Build history of the part. All positions in model axes, mm. Face numbers are marked on the shaded views. A direction names the side the tool comes from. Give positions to 0.01 mm unless a question says otherwise; leave off trailing zeros. Order: outer loops, then holes, each group sorted by start corner. A loop starts at its lowest first (then second) coordinate and runs counter-clockwise, first axis right, second up. Notation, with made-up numbers: (80, 83) -> (129, 83) arc R5 ccw to (129, 90) -> close; hole circle Ø8 at (19, 12). An arc over 180 degrees is marked (long way). Use a Markdown table: item, result. Add a question column.
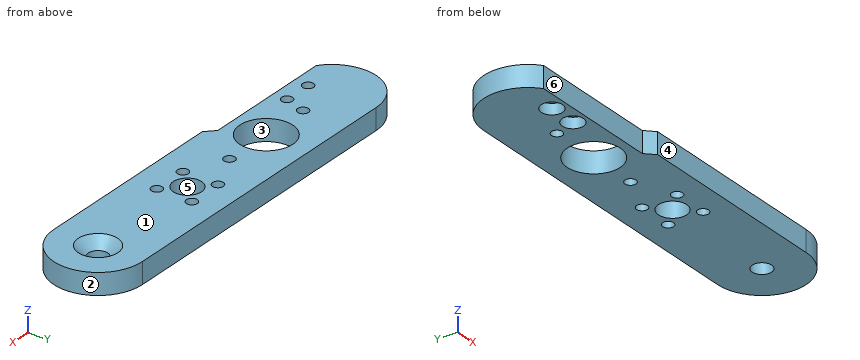
```python
from build123d import *

# Parameters (mm, degrees)
SKETCH2_R                     = 4
SKETCH2_R_2                   = 1.55
SKETCH2_R_3                   = 7.5
BOSS_EXTRUDE1_DEPTH           = 6
CSK_FOR_M5_SFHCS1_D           = 5.5
CSK_FOR_M5_SFHCS1_CSINK_D     = 11.2
CSK_FOR_M5_SFHCS1_CSINK_ANGLE = 90
SKETCH6_R                     = 1.55
CUT_EXTRUDE1_DEPTH            = 3
SKETCH7_R                     = 3
CUT_EXTRUDE2_DEPTH            = 59.49909717


with BuildPart() as part:
    # Sketch2 → Boss-Extrude1 (new body)
    with BuildSketch(Plane.XY):
        with BuildLine():
            Line((-44.569206843, 12.5), (44.430793157, 12.5))
            ThreePointArc((44.430793157, 12.5), (56.930793157, 0), (44.430793157, -12.5))
            Line((44.430793157, -12.5), (-12.069206843, -12.5))
            Line((-12.069206843, -12.5), (-14.569206843, -10))
            Line((-14.569206843, -10), (-52.069206843, -10))
            ThreePointArc((-52.069206843, -10), (-56.427748069, 3.952847075), (-44.569206843, 12.5))
        make_face()
        with Locations((10.430793157, 0)):
            Circle(SKETCH2_R, mode=Mode.SUBTRACT)
        with Locations((15.380540625, 4.949747468)):
            Circle(SKETCH2_R_2, mode=Mode.SUBTRACT)
        with Locations((15.380540625, -4.949747468)):
            Circle(SKETCH2_R_2, mode=Mode.SUBTRACT)
        with Locations((5.481045689, -4.949747468)):
            Circle(SKETCH2_R_2, mode=Mode.SUBTRACT)
        with Locations((5.481045689, 4.949747468)):
            Circle(SKETCH2_R_2, mode=Mode.SUBTRACT)
        with Locations((-19.569206843, 0)):
            Circle(SKETCH2_R_3, mode=Mode.SUBTRACT)
        with Locations((-5.569206843, 0)):
            Circle(SKETCH2_R_2, mode=Mode.SUBTRACT)
        with Locations((-33.569206843, 0)):
            Circle(SKETCH2_R_2, mode=Mode.SUBTRACT)
    extrude(amount=BOSS_EXTRUDE1_DEPTH)

    # CSK for M5 SFHCS1 (through all)
    with Locations(Plane(origin=(44.430793157, 0, 6), x_dir=(1, 0, 0), z_dir=(0, 0, 1))):
        with Locations((0, 0)):
            CounterSinkHole(CSK_FOR_M5_SFHCS1_D / 2, CSK_FOR_M5_SFHCS1_CSINK_D / 2, counter_sink_angle=CSK_FOR_M5_SFHCS1_CSINK_ANGLE)

    # Sketch6 → Cut-Extrude1 (cut)
    with BuildSketch(Plane.XY.offset(6)):
        with Locations((-35.569206843, -6)):
            Circle(SKETCH6_R)
        with Locations((-43.569206843, -6)):
            Circle(SKETCH6_R)
    extrude(amount=-CUT_EXTRUDE1_DEPTH, mode=Mode.SUBTRACT)

    # Sketch7 → Cut-Extrude2 (cut, through all)
    with BuildSketch(Plane.XY.offset(3)):
        with Locations((-35.569206843, -6)):
            Circle(SKETCH7_R)
        with Locations((-43.569206843, -6)):
            Circle(SKETCH7_R)
    extrude(amount=-CUT_EXTRUDE2_DEPTH, mode=Mode.SUBTRACT)


solid = part.part
```
(1) Wall check: probe 1 along X at (y, z) = (1.25, 5.25); probe 2 along X at (y, z) = (1, 4.55); probe 3 along Y at (x, z) = (12.5, 4.1). Give the ranges that are in metal, low to high.
(2) Mould opens along Y. For the marked faces 1, 2, 3 and 4 say: released by +Y, released by -Y, zero draft, split by the parting line, or undercut.
(3) Band-saw the part on D-D on y = 10.5. Give the cut face in (x, z), plus the area to 3 significant figures.
(4) Pin check, flat tips, straight feed: pin 1 Ø3 at (x, y) = (-44.5, -5) entering from -Z; pin 2 Ø1.8 at (x, z) = (-27.5, 3.5) entering from -Y. Stop position of each tip, or through.
(5) Band-saw the part on B-B on x = 11.5. Give the cut face in (y, z).
(6) Band-saw the part on A-A on y = 0. Give the cut face in (x, z), plus the area to 3 significant figures.
(7) Tool access for the marked faces 5 and 6: list every direction of +Z, -Z, +X, -X, +Y, -Y with a clear straight run to the whole face (end or side of a thin tool).
(8) Band-saw the part on C-C on z = 4.2. State how many separate pieces and enclosed holes the cut face has, plus the area to 3 significant figures.
Response:
| question | item | result |
|---|---|---|
| 1 | probe 1 | x = -57.01 to -34.49, -32.65 to -26.96, -12.17 to -6.49, -4.65 to 6.63, 14.23 to 39.74, 49.12 to 56.87 |
| 1 | probe 2 | x = -57.03 to -34.75, -32.38 to -27, -12.14 to -6.75, -4.38 to 6.56, 14.3 to 40.4, 48.46 to 56.89 |
| 1 | probe 3 | y = -12.5 to -3.42, 3.42 to 12.5 |
| 2 | face 1 | zero draft |
| 2 | face 2 | split by the parting line |
| 2 | face 3 | undercut |
| 2 | face 4 | released by -Y |
| 3 | outline | (-51.35, 0) -> (51.21, 0) -> (51.21, 6) -> (-51.35, 6) -> close |
| 3 | area | 615 mm² |
| 4 | pin 1 | stops at z = 3 |
| 4 | pin 2 | stops at y = -10 |
| 5 | outline | (-12.5, 0) -> (-3.85, 0) -> (-3.85, 6) -> (-12.5, 6) -> close; (3.85, 0) -> (12.5, 0) -> (12.5, 6) -> (3.85, 6) -> close |
| 6 | outline | (-57.07, 0) -> (-35.12, 0) -> (-35.12, 6) -> (-57.07, 6) -> close; (-32.02, 0) -> (-27.07, 0) -> (-27.07, 6) -> (-32.02, 6) -> close; (-12.07, 0) -> (-7.12, 0) -> (-7.12, 6) -> (-12.07, 6) -> close; (-4.02, 0) -> (6.43, 0) -> (6.43, 6) -> (-4.02, 6) -> close; (14.43, 0) -> (41.68, 0) -> (41.68, 3.15) -> (38.83, 6) -> (14.43, 6) -> close; (47.18, 0) -> (56.93, 0) -> (56.93, 6) -> (50.03, 6) -> (47.18, 3.15) -> close |
| 6 | area | 468 mm² |
| 7 | face 5 | +Z, -Z |
| 7 | face 6 | +Z, -Z, -X, -Y |
| 8 | separate pieces | 1 |
| 8 | enclosed holes | 11 |
| 8 | area | 2,290 mm² |
